The model under review builds one solid part; all positions refer to its coordinate system, in mm. Coordinates: 2 decimals unless noted, no trailing zeros. Loops run counter-clockwise (first coordinate to the right, second up) from the corner with the lowest first, then second, coordinate; pieces in that order, holes last. Notation, with made-up numbers: M 41,89.25 L 63,89.25 A23 cw 63,113.25 Z; hole C 48,0.25 d9. An arc over 180 degrees is marked long. Return JSON: item names as keys, results as strings.
```python
from build123d import *

# Parameters (mm, degrees)
F0_R     = 19.4977351631
F1_DEPTH = 22.5
F2_R     = 10


with BuildPart() as f1:
    # F0 (on Front) → F1 (new body, symmetric)
    with BuildSketch(Plane.XZ):
        with BuildLine():
            Line((-23.9709949473, -32.5), (23.9709949473, -32.5))
            Line((23.9709949473, -32.5), (23.9709949473, 32.5))
            ThreePointArc((23.9709949473, 32.5), (0, 56.4709949473), (-23.9709949473, 32.5))
            Line((-23.9709949473, 32.5), (-23.9709949473, -32.5))
        make_face()
        with Locations((0, 32.5)):
            Circle(F0_R, mode=Mode.SUBTRACT)
        with Locations((0, 32.5)):
            Circle(F0_R)
    extrude(amount=F1_DEPTH, both=True)

    # F2
    f2_edges = [f1.edges().sort_by_distance(p)[0] for p in [
        (0, -22.5, -32.5),
        (-23.970995, -22.5, 0),
        (23.970995, 0, -32.5),
        (-23.970995, 0, -32.5),
        (23.970995, 22.5, 0),
        (0, 22.5, -32.5),
    ]]
    fillet(f2_edges, radius=F2_R)


solid = f1.part
```
1. Insertion check: pin 1 Ø4 at (x, z) = (14.5, 37) entering from +Y; pin 2 Ø10 at (x, y) = (-8.5, 18) entering from -Z; pin 3 Ø1 at (x, y) = (19, -2) entering from -Z; pin 4 Ø5 at (x, y) = (6.5, -0.5) entering from +Z. Each pin has a flat end and moves straight along its axis. Give the tip position at first contact, or say it passes through.
Check values:
{"pin 1": "y = 22.5", "pin 2": "z = -32.49", "pin 3": "z = -31.42", "pin 4": "z = 56.13"}
2. Add section D-D on y = -19. Give the boundary of the cut face in (x, z).
Check values:
{"outline": "M -21.57,-22.5 A7.6 ccw -13.97,-30.1 L 13.97,-30.1 A7.6 ccw 21.57,-22.5 L 21.57,32.5 A21.57 ccw -21.57,32.5 Z"}
3. Add section B-B on x = 0. Give the boundary of the cut face in (y, z).
Check values:
{"outline": "M -22.5,-22.5 A10 ccw -12.5,-32.5 L 12.5,-32.5 A10 ccw 22.5,-22.5 L 22.5,46.47 A10 ccw 12.5,56.47 L -12.5,56.47 A10 ccw -22.5,46.47 Z"}
4. Add section A-A on z = -14. Give the boundary of the cut face in (x, y).
Check values:
{"outline": "M -23.97,-12.5 A10 ccw -13.97,-22.5 L 13.97,-22.5 A10 ccw 23.97,-12.5 L 23.97,12.5 A10 ccw 13.97,22.5 L -13.97,22.5 A10 ccw -23.97,12.5 Z"}
5. To check wall thickness, follow line 1 (Y direction, x = 13, z = 38); line 2 (X direction, y = 19, z = 12.5); line 3 (Z direction, x = -20, y = -4.5). State the ranges of each line that lie inside material, in increasing order.
Check values:
{"line 1": "-22.5 to 22.5", "line 2": "-21.57 to 21.57", "line 3": "-30.48 to 45.71"}
6. Add section C-C on y = -6. Give the boundary of the cut face in (x, z), plus the area to 3 significant figures.
Check values:
{"outline": "M -23.97,-22.5 A10 ccw -13.97,-32.5 L 13.97,-32.5 A10 ccw 23.97,-22.5 L 23.97,32.5 A23.97 ccw -23.97,32.5 Z", "area": "3,980 mm²"}
